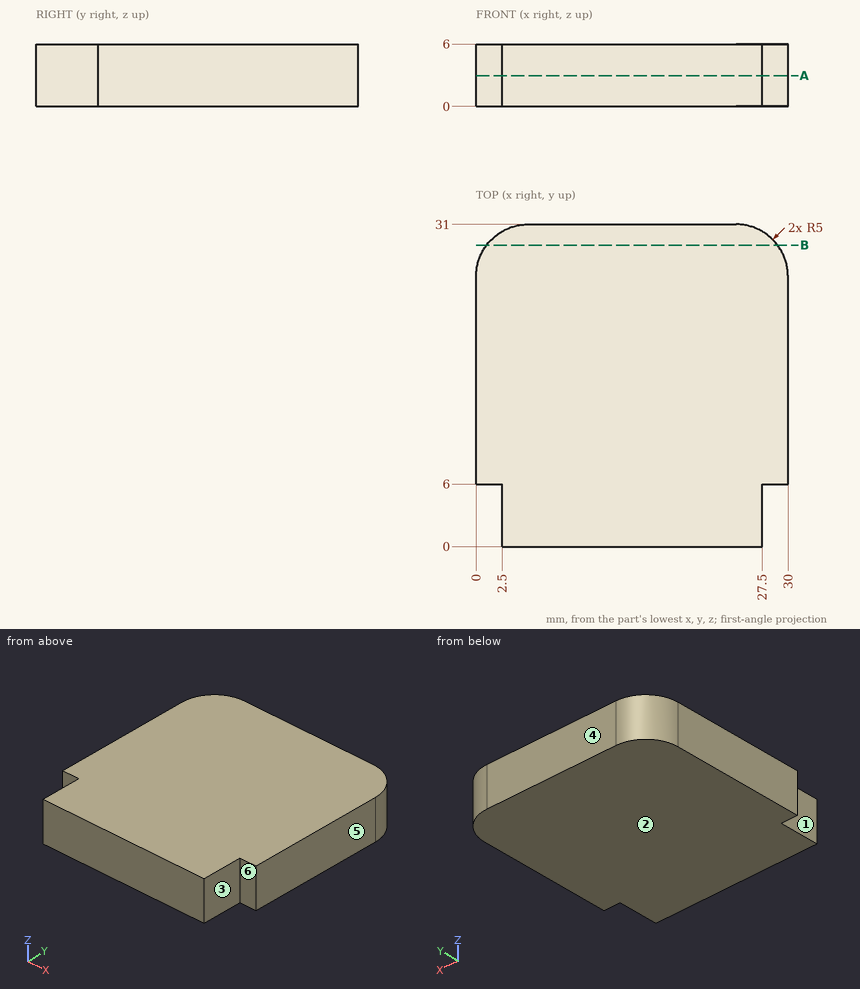
Design review of the part shown in the three views and the two pictorial views. Dimensions are in mm from the part's minimum x, y and z. A direction names the side the tool comes from. Round coordinates to 2 decimals unless told otherwise and drop trailing zeros. Order: outer loops, then holes, each group sorted by start corner. A loop starts at its lowest first (then second) coordinate and runs counter-clockwise, first axis right, second up. Notation, with made-up numbers: (70, 37) -> (76, 37) arc R27 cw to (76, 67) -> close; hole circle Ø4 at (51, 45.25). An arc over 180 degrees is marked (long way). Write item = value, one per line. Start each with the question number.
1) Tool access review of the marked faces 1, 2 and 3: name each direction out of +Z, -Z, +X, -X, +Y, -Y from which nothing blocks a thin tool from reaching the whole face with its end or side.
2) To check wall thickness, follow line 1 (Y direction, x = 2, z = 1.6); line 2 (X direction, y = 29.5, z = 4.65); line 3 (Y direction, x = 26.5, z = 2.5). State the ranges of each line that lie inside material, in increasing order. Write a range as from..to.
3) Insertion check: pin 1 (3 mm diameter, centred on y = 22, z = 0.5, fed in from -X); pin 2 (3 mm diameter, centred on y = 2.5, z = 3, fed in from +X); pin 3 (0.8 mm diameter, centred on x = 1, z = 4, fed in from -Y). Each pin has a flat end and moves straight along its axis. Give the tip position at first contact, or say it passes through.
4) The part is to be moulded in two halves that separate along Y. For the marked faces 4, 5 and 6, say which applies: +Y half, -Y half, draft (parallel to the pull), parting line (faces both ways), or undercut.
5) Take a section at B-B on y = 29. State the section outline as (x, z) points, plus the area to 3 significant figures.
6) Take a section at A-A on z = 2.95. State the section outline as (x, y) points, plus the area to 3 significant figures.
Verdict:
q1.face_1 = +Z, -Z, -X, -Y
q1.face_2 = -Z, +X, -X, +Y, -Y
q1.face_3 = +Z, -Z, +X, -Y
q2.line_1 = 6..30
q2.line_2 = 1.43..28.57
q2.line_3 = 0..30.77
q3.pin_1 = 0
q3.pin_2 = 27.5
q3.pin_3 = 6
q4.face_4 = +Y half
q4.face_5 = draft
q4.face_6 = -Y half
q5.outline = (1, 0) -> (29, 0) -> (29, 6) -> (1, 6) -> close
q5.area = 168 mm2
q6.outline = (0, 6) -> (2.5, 6) -> (2.5, 0) -> (27.5, 0) -> (27.5, 6) -> (30, 6) -> (30, 26) arc R5 ccw to (25, 31) -> (5, 31) arc R5 ccw to (0, 26) -> close
q6.area = 889 mm2
